```python
from build123d import *

# Parameters (mm, degrees)
SKETCH_1_R      = 2.15
EXTRUDE_1_DEPTH = 4
FILLET_1_R      = 0.2
FILLET_2_R      = 2
FILLET_3_R      = 2
FILLET_4_R      = 8.5
SKETCH_2_R      = 1.525
EXTRUDE_2_DEPTH = 4
FILLET_5_R      = 2


with BuildPart() as part:
    # 草图1 → 凸台-拉伸1 (new body)
    with BuildSketch(Plane.XY):
        with BuildLine():
            Line((-52, 8.75), (-52, 30))
            Line((-52, 30), (-47.54, 30))
            ThreePointArc((-47.54, 30), (-44.004466094, 31.464466094), (-42.54, 35))
            Line((-42.54, 35), (-42.54, 37.5))
            ThreePointArc((-42.54, 37.5), (-38.982425028, 42.287422066), (-33.372235985, 40.262198963))
            ThreePointArc((-33.372235985, 40.262198963), (-30.171244586, 38.118753147), (-26.396349665, 38.887436588))
            ThreePointArc((-26.396349665, 38.887436588), (0, 47), (26.396349665, 38.887436588))
            ThreePointArc((26.396349665, 38.887436588), (30.171244586, 38.118753147), (33.372235985, 40.262198963))
            ThreePointArc((33.372235985, 40.262198963), (38.674773042, 42.369526686), (42.499484755, 38.135225128))
            Line((42.499484755, 38.135225128), (46.619156699, 5.971116201))
            ThreePointArc((46.619156699, 5.971116201), (47, 0), (46.619156699, -5.971116201))
            Line((46.619156699, -5.971116201), (42.499484755, -38.135225128))
            ThreePointArc((42.499484755, -38.135225128), (38.674773042, -42.369526686), (33.372235985, -40.262198963))
            ThreePointArc((33.372235985, -40.262198963), (30.171244586, -38.118753147), (26.396349665, -38.887436588))
            ThreePointArc((26.396349665, -38.887436588), (0, -47), (-26.396349665, -38.887436588))
            ThreePointArc((-26.396349665, -38.887436588), (-30.171244586, -38.118753147), (-33.372235985, -40.262198963))
            ThreePointArc((-33.372235985, -40.262198963), (-38.982425028, -42.287422066), (-42.54, -37.5))
            Line((-42.54, -37.5), (-42.54, -35))
            ThreePointArc((-42.54, -35), (-44.004466094, -31.464466094), (-47.54, -30))
            Line((-47.54, -30), (-52, -30))
            Line((-52, -30), (-52, -8.75))
            Line((-52, -8.75), (-40.055430343, -8.75))
            ThreePointArc((-40.055430343, -8.75), (40.804364959, -4.000475011), (-37.593370285, 16.362717092))
            ThreePointArc((-37.593370285, 16.362717092), (-29.005163231, 12.290176631), (-21.585495377, 6.349518825))
            ThreePointArc((-21.585495377, 6.349518825), (-22.451945258, -1.469746278), (-20.573530425, -9.10932741))
            ThreePointArc((-20.573530425, -9.10932741), (-28.44850534, 1.855840669), (-40.055430343, 8.75))
            Line((-40.055430343, 8.75), (-52, 8.75))
        make_face()
        with Locations((-37.54, 37.5)):
            Circle(SKETCH_1_R, mode=Mode.SUBTRACT)
        with Locations((-37.54, -37.5)):
            Circle(SKETCH_1_R, mode=Mode.SUBTRACT)
        with Locations((37.54, -37.5)):
            Circle(SKETCH_1_R, mode=Mode.SUBTRACT)
        with Locations((37.54, 37.5)):
            Circle(SKETCH_1_R, mode=Mode.SUBTRACT)
    extrude(amount=EXTRUDE_1_DEPTH)

    # 圆角1
    fillet_1_edges = [part.edges().sort_by_distance(p)[0] for p in [
        (-20.573530425, -9.10932741, 2),
    ]]
    fillet(fillet_1_edges, radius=FILLET_1_R)

    # 圆角2
    fillet_2_edges = [part.edges().sort_by_distance(p)[0] for p in [
        (-21.585495377, 6.349518825, 2),
    ]]
    fillet(fillet_2_edges, radius=FILLET_2_R)

    # 圆角3
    fillet_3_edges = [part.edges().sort_by_distance(p)[0] for p in [
        (-37.593370285, 16.362717092, 2),
    ]]
    fillet(fillet_3_edges, radius=FILLET_3_R)

    # 圆角4
    fillet_4_edges = [part.edges().sort_by_distance(p)[0] for p in [
        (-40.055430343, 8.75, 2),
    ]]
    fillet(fillet_4_edges, radius=FILLET_4_R)

    # 草图2 → 凸台-拉伸2 (add)
    # profile 1 of 2: a face of its own
    with BuildSketch(Plane(origin=(0, 0, 0), x_dir=(-1, 0, 0), z_dir=(0, 0, -1))):
        with BuildLine():
            Line((1.733082495, -49.911702088), (1.733082495, -46.968036206))
            ThreePointArc((1.733082495, -46.968036206), (4.894207665, -46.744483432), (8.033082495, -46.308418086))
            Line((8.033082495, -46.308418086), (8.033082495, -49.911702088))
            ThreePointArc((8.033082495, -49.911702088), (4.883082495, -53.061702088), (1.733082495, -49.911702088))
        make_face()
        with Locations((4.883082495, -49.911702088)):
            Circle(SKETCH_2_R, mode=Mode.SUBTRACT)
    # profile 2 of 2: a face of its own
    with BuildSketch(Plane(origin=(0, 0, 0), x_dir=(-1, 0, 0), z_dir=(0, 0, -1))):
        with BuildLine():
            Line((21.234134605, -45.541810763), (19.676083646, -42.683155136))
            ThreePointArc((19.676083646, -42.683155136), (22.492522433, -41.268467801), (25.207814436, -39.668200001))
            Line((25.207814436, -39.668200001), (26.765865395, -42.526855629))
            ThreePointArc((26.765865395, -42.526855629), (25.507477567, -46.800198591), (21.234134605, -45.541810763))
        make_face()
        with Locations((24, -44.034333196)):
            Circle(SKETCH_2_R, mode=Mode.SUBTRACT)
    extrude(amount=-EXTRUDE_2_DEPTH)

    # 圆角5
    fillet_5_edges = [part.edges().sort_by_distance(p)[0] for p in [
        (-1.733082495, -46.968036206, 2),
        (-19.676083646, -42.683155136, 2),
        (-25.207814436, -39.668200001, 2),
        (-8.033082495, -46.308418086, 2),
    ]]
    fillet(fillet_5_edges, radius=FILLET_5_R)


solid = part.part
```
Geometry check sheet. Reference: the model listing, model coordinates, mm. A direction names the side the tool comes from. Round coordinates to 2 decimals unless told otherwise and drop trailing zeros. Order: outer loops, then holes, each group sorted by start corner. A loop starts at its lowest first (then second) coordinate and runs counter-clockwise, first axis right, second up. Notation, with made-up numbers: (40, -7.5) - (77, -7.5) arc R17 ccw to (77, 1.5) - close; hole circle Ø9 at (-24, -32.75). An arc over 180 degrees is marked (long way). Use a Markdown table: item, result. Add a question column.
1) Section check A-A (y = -31.5). Record the cut outline in (x, z), then the cut area to 3 significant figures.
2) Set-up check for faces 1 (the flat face through (-50, 30, 2)), 2 (the cylindrical face through (-13.83, -44.92, 1.97)), 3 (the flat face through (-50, -30, 2)): record each of +Z, -Z, +X, -X, +Y, -Y from which the full face is reachable in a straight line by a thin tool's end or side.
3) Thickness scan on line 1 along Y through (x, z) = (-37.54, 1.35); line 2 along Y through (x, z) = (37.54, 1); line 3 along Y through (x, z) = (-3.5, 1.25). Record the ranges inside material, lowest first.
4) Section check B-B (x = -4.5). Record the cut outline in (y, z), then the cut area to 3 significant figures.
5) Section check D-D (x = 28). Record the cut outline in (y, z), then the cut area to 3 significant figures.
6) Gauge pin test, flat ends, axial feed: P1, Ø2, axis at x = -49.5, z = 3, coming from the -Y side; P2, Ø2, axis at y = -48.5, z = 2.5, coming from the -X side; P3, Ø0.8, axis at y = -36, z = 2, coming from the -X side. Record the tip position at first contact, or that the pin passes through.
7) Mould release check, pull along Y, two halves, no side actions. Record for faces 4 (the flat face through (-24, 1, 4)), 5 (the flat face through (44.588, -21.828, 1.972)), 6 (the cylindrical face through (-28.704, 12.1, 1.972)): released by +Y, released by -Y, zero draft, split by the parting line, or undercut.
8) Section check C-C (x = -24). Record the cut outline in (y, z).
Established:
| question | item | result |
|---|---|---|
| 1 | outline | (-43.97, 0) - (-26.24, 0) - (-26.24, 4) - (-43.97, 4) - close; (26.24, 0) - (43.35, 0) - (43.35, 4) - (26.24, 4) - close |
| 1 | area | 139 mm2 |
| 2 | face 1 | +Z, -Z, -X, +Y |
| 2 | face 2 | +Z, -Z, -Y |
| 2 | face 3 | +Z, -Z, -X, -Y |
| 3 | line 1 | -42.5 to -39.65, -35.35 to -16.48, 7.77 to 35.35, 39.65 to 42.5 |
| 3 | line 2 | -42.5 to -39.65, -35.35 to -16.48, 16.48 to 35.35, 39.65 to 42.5 |
| 3 | line 3 | -52.74 to -50.55, -49.27 to -40.85, 40.85 to 46.87 |
| 4 | outline | (-53.04, 0) - (-51.39, 0) - (-51.39, 4) - (-53.04, 4) - close; (-48.44, 0) - (-40.75, 0) - (-40.75, 4) - (-48.44, 4) - close; (40.75, 0) - (46.78, 0) - (46.78, 4) - (40.75, 4) - close |
| 4 | area | 61.5 mm2 |
| 5 | outline | (-38.17, 0) - (-29.95, 0) - (-29.95, 4) - (-38.17, 4) - close; (29.95, 0) - (38.17, 0) - (38.17, 4) - (29.95, 4) - close |
| 5 | area | 65.8 mm2 |
| 6 | P1 | y = -30 |
| 6 | P2 | x = -8.09 |
| 6 | P3 | x = -42.54 |
| 7 | face 4 | zero draft |
| 7 | face 5 | released by -Y |
| 7 | face 6 | undercut |
| 8 | outline | (-47.18, 0) - (-45.56, 0) - (-45.56, 4) - (-47.18, 4) - close; (-42.51, 0) - (-33.24, 0) - (-33.24, 4) - (-42.51, 4) - close; (-3.14, 0) - (8.6, 0) - (8.6, 4) - (-3.14, 4) - close; (33.24, 0) - (40.41, 0) - (40.41, 4) - (33.24, 4) - close |
